Could you check a few things on this model? Use its own coordinates, in mm. Face numbers are marked on the shaded views. Give positions to 0.01 mm unless a question says otherwise; leave off trailing zeros. Loops run counter-clockwise (first coordinate to the right, second up) from the corner with the lowest first, then second, coordinate; pieces in that order, holes last.
1. Imagine slicing it at A-A (z = 4). List the corners of the cut face in (x, y) for me.
2. Imagine slicing it at C-C (y = 3.05). List the corners of the cut face in (x, z) for me.
3. Imagine slicing it at B-B (y = 0.6). Count the separate pieces of the cut face and the enclosed holes in it, plus the area to 3 significant figures.
4. Thinking about a two-plate mould opening in Z: for the marked faces 1, 2 and 3, which applies, +Z half, -Z half, draft (parallel to the pull), parting line (faces both ways), or undercut?
5. I need wall thicknesses on line 1 along Z through (x, y) = (0, 1.7); line 2 along Y through (x, z) = (2, -5); line 3 along Z through (x, y) = (-2.25, 1.85). Which ranges of each line are inside material? Lowest first, please.
6. For P1, Ø1.7, axis at x = -0.5, z = 7, coming from the +Y side, with a flat end and sliding along its axis, tell me the tip position at first contact or that it passes through.
Autodesk Fusion 360 part; units mm, degrees
sketch "草图1" plane through (0, 0, 0) normal (0, 1, 0) x (1, 0, 0)
  circle A0 centre (0, 0) radius 3.5
  line L0 (0, 0) -> (0, -16)
  line L1 (0, 0) -> (0, 16)
  circle A1 centre (0, -16) radius 2
  circle A2 centre (0, 16) radius 2
  line L2 (0, 16) -> (6, 16)
  line L3 (6, 16) -> (-7, 16)
  line L4 (2, 16) -> (2.8777, 2.0488)
  line L5 (2, 16) -> (15.9788, 16) construction
  line L6 (-2, 16) -> (-2.8733, 2.1192)
  line L7 (-2, 16) -> (11.9083, 16) construction
  line L8 (0, -16) -> (5, -16)
  line L9 (5, -16) -> (-6, -16)
  line L10 (2, -16) -> (2.8901, -1.8524)
  line L11 (2, -16) -> (16.1756, -16) construction
  line L12 (-2, -16) -> (-2.8817, -1.9865)
  line L13 (-2, -16) -> (12.0412, -16) construction
  line L14 (2.8777, 2.0488) -> (2.8885, 1.8784)
  line L15 (-2.8733, 2.1192) -> (-2.9, 1.6952)
  dimension "d1" = 7
  dimension "d2" = 16
  dimension "d3" = 16
  dimension "d4" = 4
  dimension "d5" = 4
  dimension "d6" = 86.4
  dimension "d7" = 93.6
  dimension "d8" = 13.9083
  dimension "d9" = 86.4
  dimension "d10" = 93.6
extrude "拉伸1" add sketch "草图1" along normal blind 1.5
sketch "草图2" plane through (0, 1.5, 0) normal (0, 1, 0) x (-1, 0, 0)
  arc A0 (-2, -16) -> (2, -16) centre (0, -16) ccw
  line L0 (2, -16) -> (2.8817, -1.9865)
  arc A1 (2.8817, -1.9865) -> (2.8817, 1.9865) centre (0, 0) ccw
  line L1 (2.8817, 1.9865) -> (2, 16)
  arc A2 (2, 16) -> (-2, 16) centre (0, 16) ccw
  line L2 (-2, 16) -> (-2.8817, 1.9865)
  arc A3 (-2.8817, 1.9865) -> (-2.8817, -1.9865) centre (0, 0) ccw
  line L3 (-2.8817, -1.9865) -> (-2, -16)
  circle A4 centre (0, 0) radius 3.5
extrude "拉伸2" add sketch "草图2" along normal blind 2 contours A1 A3 A4
sketch "草图3" plane through (0, 1.5, 0) normal (0, 1, 0) x (-1, 0, 0)
  arc A0 (-2.8817, -1.9865) -> (2.8817, -1.9865) centre (0, 0) ccw
  line L0 (-2.8817, -1.9865) -> (-2, -16)
  arc A1 (-2, -16) -> (2, -16) centre (0, -16) ccw
  line L1 (2, -16) -> (2.8817, -1.9865)
  line L2 (0, -4) -> (0, -16.75)
  line L3 (0, -16.75) -> (0, -14.2)
  line L4 (0, -14.2) -> (0, -11.65)
  line L5 (0, -11.65) -> (0, -9.1)
  line L6 (0, -9.1) -> (0, -6.55)
  circle A2 centre (0, -4) radius 0.45
  circle A3 centre (0, -16.75) radius 0.45
  circle A4 centre (0, -14.2) radius 0.45
  circle A5 centre (0, -11.65) radius 0.45
  circle A6 centre (0, -9.1) radius 0.45
  circle A7 centre (0, -6.55) radius 0.45
  line L7 (-8.6176, 0) -> (8, 0)
  circle A8 centre (0, 16.75) radius 0.45
  circle A9 centre (0, 14.2) radius 0.45
  circle A10 centre (0, 11.65) radius 0.45
  circle A11 centre (0, 9.1) radius 0.45
  circle A12 centre (0, 6.55) radius 0.45
  circle A13 centre (0, 4) radius 0.45
  dimension "d26" = 12.75
  dimension "d28" = 2.55
  dimension "d29" = 2.55
  dimension "d30" = 2.55
  dimension "d31" = 2.55
  dimension "d32" = 0.9
  dimension "d33" = 0.9
  dimension "d34" = 0.9
  dimension "d35" = 0.9
  dimension "d36" = 0.9
  dimension "d37" = 0.9
extrude "拉伸3" cut sketch "草图3" against normal blind 8 contours A3 | L2 L3 L4 A4 | L2 L3 L4 A4 | L2 L4 L5 A5 | L2 L4 L5 A5 | L2 L5 L6 A6 | L2 L5 L6 A6 | L2 L6 A7 | L2 L6 A7 | A2 | A8 | A9 | A10 | A11 | A12 | A13
sketch "草图4" plane through (0, 0, 0) normal (0, -1, 0) x (1, 0, 0)
  circle A0 centre (0, 11.65) radius 0.45
  circle A1 centre (0, -4) radius 0.45
  circle A2 centre (0, -14.2) radius 0.45
  circle A3 centre (0, -11.65) radius 0.45
  circle A4 centre (0, 4) radius 0.45
  circle A5 centre (0, 14.2) radius 0.45
  circle A6 centre (0, 9.1) radius 0.45
  circle A7 centre (0, -6.55) radius 0.45
  circle A8 centre (0, -16.75) radius 0.45
  circle A9 centre (0, -9.1) radius 0.45
  circle A10 centre (0, 6.55) radius 0.45
  circle A11 centre (0, 16.75) radius 0.45
  arc A12 (-2, -16) -> (2, -16) centre (0, -16) ccw
  line L0 (2, -16) -> (2.8817, -1.9865)
  arc A13 (2.8817, -1.9865) -> (2.8817, 1.9865) centre (0, 0) ccw
  line L1 (2.8817, 1.9865) -> (2, 16)
  arc A14 (2, 16) -> (-2, 16) centre (0, 16) ccw
  line L2 (-2, 16) -> (-2.8817, 1.9865)
  arc A15 (-2.8817, 1.9865) -> (-2.8817, -1.9865) centre (0, 0) ccw
  line L3 (-2.8817, -1.9865) -> (-2, -16)
  circle A16 centre (0, 0) radius 2.3
  dimension "d40" = 4.6
extrude "拉伸4" cut sketch "草图4" against normal blind 1 contours A16
sketch "草图5" plane through (0, 1, 0) normal (0, -1, 0) x (1, 0, 0)
  circle A0 centre (0, 0) radius 2.3
  circle A1 centre (0, 0) radius 1.25
  dimension "d43" = 2.5
extrude "拉伸5" cut sketch "草图5" against normal blind 10 contours A1
sketch "草图6" plane through (0, 3.5, 0) normal (0, 1, 0) x (-1, 0, 0)
  circle A0 centre (0, 0) radius 1.25
  circle A1 centre (0, 0) radius 3.5
  circle A2 centre (0, 0) radius 2.5
  dimension "d46" = 5
extrude "拉伸6" cut sketch "草图6" against normal blind 2 contours A2
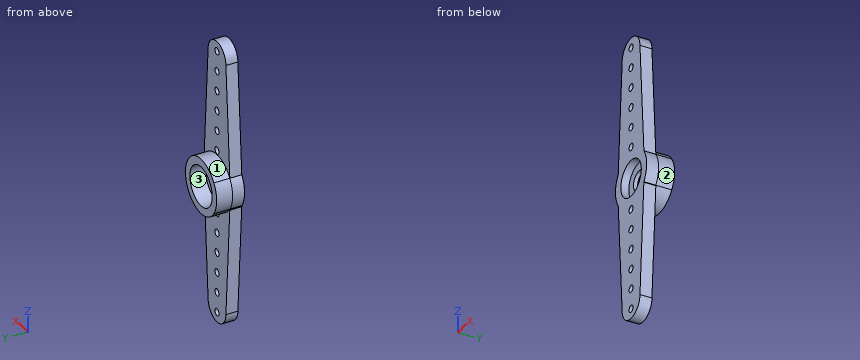
Derived:
1. outline: (-2.76, 0) - (-0.45, 0) - (-0.45, 1.5) - (-2.76, 1.5) - close; (0.45, 0) - (2.75, 0) - (2.75, 1.5) - (0.45, 1.5) - close
2. outline: (-2.88, -1.99) arc R3.5 ccw to (2.88, -1.99) arc R3.5 ccw (long way) to start; hole circle Ø5 at (0, 0)
3. separate pieces: 1
3. enclosed holes: 13
3. area: 151 mm2
4. face 1: +Z half
4. face 2: parting line
4. face 3: undercut
5. line 1: z = -3.5 to -2.5, 2.5 to 3.5
5. line 2: y = 0 to 1.5
5. line 3: z = -2.68 to -1.09, 1.09 to 2.68
6. P1: stops at y = 1.5
